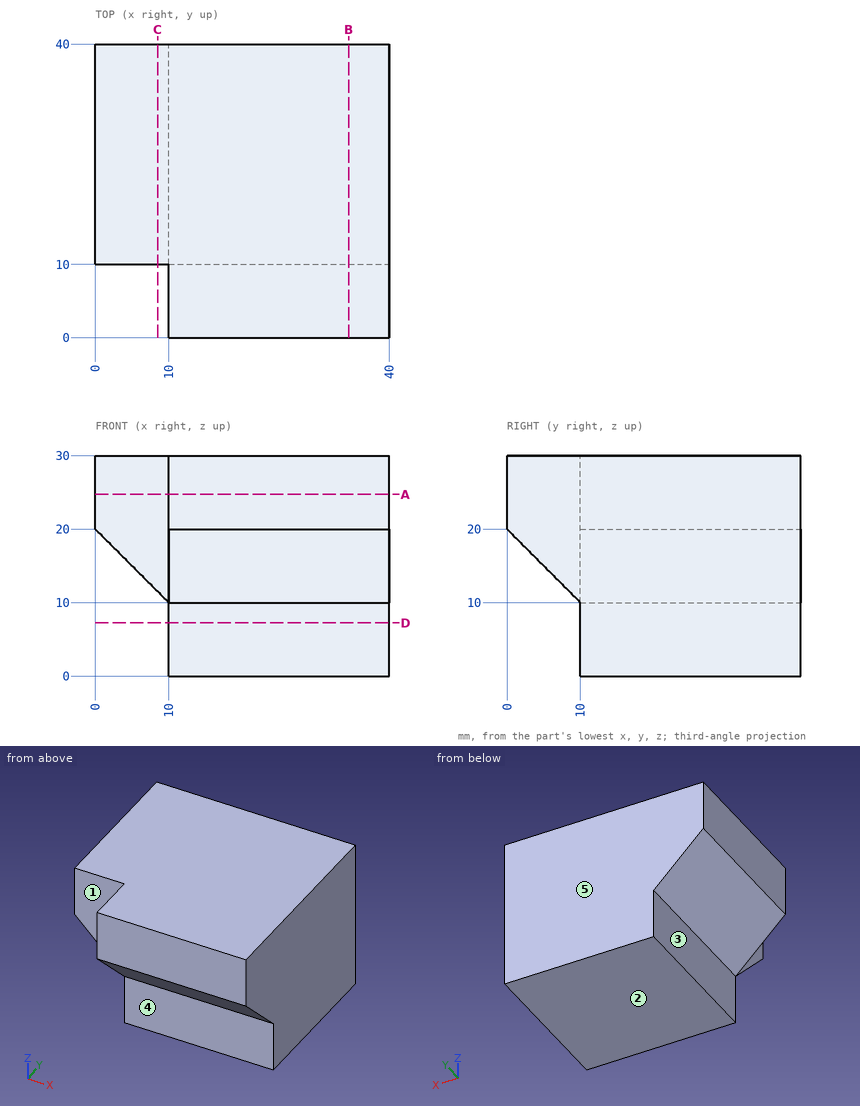
The drawing under review shows one solid part. Ordinate dimensions are in mm from its lowest x, y, z. A direction names the side the tool comes from. Round coordinates to 2 decimals unless told otherwise and drop trailing zeros. Write each loop counter-clockwise with the first axis right and the second up, starting at its lowest first coordinate (ties: lowest second). Pieces come first, ordered by that corner, then holes. Notation, with made-up numbers: (-10.75, 56) - (27.25, 56) arc R20 cw to (27.25, 66) - close; hole circle Ø5 at (-33.75, 81.5). An arc over 180 degrees is marked (long way). Use a Markdown table: item, result. Add a question column.
1. For the marked faces 1, 2, 3, 4 and 5, list the 3-axis set-ups (+Z, -Z, +X, -X, +Y, -Y) from which the entire face can be reached by the end or side of a thin tool; tool diameter is ignored.
2. Clearance check with flat-ended pins moving along their axes: pin 1 (4 mm diameter, centred on x = 28, y = 7.5, fed in from -Z); pin 2 (8 mm diameter, centred on y = 5, z = 22, fed in from -X); pin 3 (6 mm diameter, centred on y = 22, z = 12.5, fed in from -X); pin 4 (12 mm diameter, centred on x = 29.5, y = 24.5, fed in from -Z). State where each tip first meets the part, or that it passes through.
3. We need section B-B (x = 34.5). State the section outline as (y, z) points.
4. We need section D-D (z = 7.25). State the section outline as (x, y) points.
5. We need section A-A (z = 24.75). State the section outline as (x, y) points.
6. Wall thickness on probe 1 along X at (y, z) = (23.5, 8.25); probe 2 along Z at (x, y) = (8, 21): over which ranges is each line inside the solid? List them lowest first.
7. We need section C-C (x = 8.5). State the section outline as (y, z) points, then the cut area to 3 significant figures.
Output:
| question | item | result |
|---|---|---|
| 1 | face 1 | +Z, -Z, -X, -Y |
| 1 | face 2 | -Z, +X, -X, +Y, -Y |
| 1 | face 3 | -Z, -X, +Y, -Y |
| 1 | face 4 | -Z, +X, -X, -Y |
| 1 | face 5 | +Z, -Z, +X, -X, +Y |
| 2 | pin 1 | stops at z = 10.5 |
| 2 | pin 2 | stops at x = 10 |
| 2 | pin 3 | stops at x = 4.5 |
| 2 | pin 4 | stops at z = 0 |
| 3 | outline | (0, 20) - (10, 10) - (10, 0) - (40, 0) - (40, 30) - (0, 30) - close |
| 4 | outline | (10, 10) - (40, 10) - (40, 40) - (10, 40) - close |
| 5 | outline | (0, 10) - (10, 10) - (10, 0) - (40, 0) - (40, 40) - (0, 40) - close |
| 6 | probe 1 | x = 10 to 40 |
| 6 | probe 2 | z = 12 to 30 |
| 7 | outline | (10, 11.5) - (40, 11.5) - (40, 30) - (10, 30) - close |
| 7 | area | 555 mm2 |
